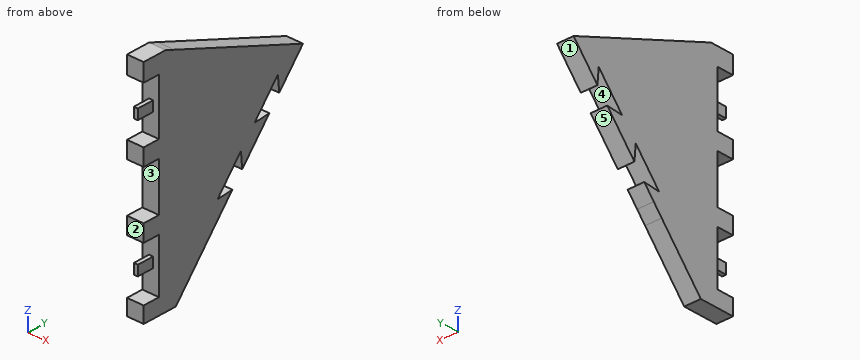
from build123d import *

# Parameters (mm, degrees)
BOSS_EXTRUDE2_DEPTH = 5
BOSS_EXTRUDE3_START = 2.05
SKETCH2_4_W         = 3
SKETCH2_4_H         = 5
BOSS_EXTRUDE3_DEPTH = 1.2


with BuildPart() as part:
    # Sketch2 → Boss-Extrude2 (new body)
    with BuildSketch(Plane(origin=(0, 0, 0), x_dir=(0, 0, -1), z_dir=(1, 0, 0))):
        Polygon((7.192857145, 5.102e-06), (12.192857145, 5.102e-06), (12.192857145, 4.998838637), (18.442857145, 4.998838637), (21.442857145, 4.998838637), (27.892857145, 4.998838637), (28.158909208, 4.998838637), (28.158909208, 0.00505468), (32.892857145, 0.00505468), (32.892857145, 10.509453346), (17.646665318, 23.302527285), (14.567046792, 25.886634054), (10.859778292, 28.997401685), (11.284525034, 24.142524207), (2.174678599, 31.786592991), (7.029556077, 32.211339733), (-3.541857238, 41.081808747), (-3.117110496, 36.226931269), (-12.226956931, 43.871000053), (-7.372079454, 44.295746795), (-16.638484456, 52.071183815), (-32.892857145, 10.00505468), (-33.983618254, 7.182177505), (-33.983618254, 0.00505468), (-32.892857145, 0.00505468), (-28.691927734, 0.00505468), (-28.691927734, 4.998838637), (-27.892857145, 4.998838637), (-21.442857145, 4.998838637), (-18.442857145, 4.998838637), (-12.192857145, 4.998838637), (-12.192857145, 4.163e-06), (-7.192857145, 4.163e-06), (-7.192857145, 5.000004163), (7.192857145, 5.000004163), align=None)
    extrude(amount=BOSS_EXTRUDE2_DEPTH)

    # Sketch2<4> → Boss-Extrude3 (add)
    with BuildSketch(Plane(origin=(0, 0, 0), x_dir=(0, 0, -1), z_dir=(1, 0, 0)).offset(BOSS_EXTRUDE3_START)):
        with Locations((19.942857145, 2.498838637)):
            Rectangle(SKETCH2_4_W, SKETCH2_4_H)
        with Locations((-19.942857145, 2.498838637)):
            Rectangle(SKETCH2_4_W, SKETCH2_4_H)
    extrude(amount=BOSS_EXTRUDE3_DEPTH)


solid = part.part
Geometry check sheet. Reference: the model listing, model coordinates, mm. Face numbers are marked on the shaded views. A direction names the side the tool comes from. Round coordinates to 2 decimals unless told otherwise and drop trailing zeros. Order: outer loops, then holes, each group sorted by start corner. A loop starts at its lowest first (then second) coordinate and runs counter-clockwise, first axis right, second up. Notation, with made-up numbers: M -1,85.25 L 56,85.25 A30 cw 56,121.25 Z; hole C -15.75,-29 d3. An arc over 180 degrees is marked long. Write each question's results on one line, items separated by ' | '. Start each with the question number.
1. Draft check along Z on the marked faces 1, 2 and 3. Enter one of: pulls with the +Z half, pulls with the -Z half, needs draft (parallel to the pull), parting line crosses it, or undercut.
2. Cross-section at A-A on z = 8.5. Record the boundary of the cut face in (x, y), plus the area to 3 significant figures.
3. Set-up check for the marked faces 4 and 5: record each of +Z, -Z, +X, -X, +Y, -Y from which the full face is reachable in a straight line by a thin tool's end or side.
4. Go/stop test with flat-tipped pins: P1, Ø1.5, axis at x = 3, z = -18, coming from the -Y side; P2, Ø0.9, axis at y = 3, z = -20, coming from the -X side; P3, Ø1.5, axis at x = 2, z = 17.5, coming from the -Y side; P4, Ø3.5, axis at y = 2, z = -20, coming from the +X side. Record where each tip stops, or that it passes through.
5. Cross-section at C-C on z = -5. Record the boundary of the cut face in (x, y).
6. Cross-section at B-B on x = 1.2. Record the boundary of the cut face in (y, z), plus the area to 3 significant figures.
7. Cross-section at D-D on y = 45. Record the boundary of the cut face in (x, z).
8. Material ranges on L1, parallel to Y at x = 4.7, z = 11.5; L2, parallel to Z at x = 2.95, y = 28.5; L3, parallel to Z at x = 3.2, y = 29.5, recorded low to high. Write a range as from..to.
Resolved:
1) face 1: pulls with the -Z half | face 2: needs draft | face 3: undercut
2) outline: M 0,0 L 5,0 L 5,40.74 L 0,40.74 Z; M 0,44.2 L 5,44.2 L 5,45.24 L 0,45.24 Z | area: 209 mm2
3) face 4: +X, -X | face 5: -Z, +X, -X, +Y
4) P1: y = 0 | P2: x = 2.05 | P3: y = 5 | P4: x = 3.25
5) outline: M 0,5 L 5,5 L 5,29.42 L 0,29.42 Z; M 0,32.03 L 5,32.03 L 5,33.91 L 0,33.91 Z
6) outline: M 0,-12.19 L 5,-12.19 L 5,-28.16 L 0.01,-28.16 L 0.01,-32.89 L 10.51,-32.89 L 29,-10.86 L 24.14,-11.28 L 31.79,-2.17 L 32.21,-7.03 L 41.08,3.54 L 36.23,3.12 L 43.87,12.23 L 44.3,7.37 L 52.07,16.64 L 7.18,33.98 L 0.01,33.98 L 0.01,28.69 L 5,28.69 L 5,12.19 L 0,12.19 L 0,7.19 L 5,7.19 L 5,-7.19 L 0,-7.19 Z | area: 1,770 mm2
7) outline: M 0,8.21 L 5,8.21 L 5,19.37 L 0,19.37 Z
8) L1: 0..43.26, 43.93..47.76 | L2: -11.45..-10.9, -6.09..25.75 | L3: -4.9..25.36
